Source: CAD feature listing. Evaluate the final solid. Frame: model axes, mm. A direction names the side the tool comes from. Round coordinates to 2 decimals unless told otherwise and drop trailing zeros. Write each loop counter-clockwise with the first axis right and the second up, starting at its lowest first coordinate (ties: lowest second). Pieces come first, ordered by that corner, then holes. Notation, with made-up numbers: M 35,-28 L 75,-28 A29 ccw 75,6 Z; hole C 20,75 d11. An arc over 180 degrees is marked long. Put each result on its own line as item: value. Start each with the question number.
```python
from build123d import *

# Parameters (mm, degrees)
F0_R     = 10.535173
F1_DEPTH = 40.894


with BuildPart() as f1:
    # F0 (on Front) → F1 (new body)
    with BuildSketch(Plane.XZ):
        with BuildLine():
            Line((-35.451322, 27.514845), (-11.27987, 27.514845))
            ThreePointArc((-11.27987, 27.514845), (-17.816037, 48.643776), (-35.141124, 62.391305))
            ThreePointArc((-35.141124, 62.391305), (-86.04097, 25.118193), (-30.793919, -5.342315))
            ThreePointArc((-30.793919, -5.342315), (-19.953258, 3.559245), (-13.152019, 15.827123))
            Line((-13.152019, 15.827123), (-42.462349, 15.827123))
            ThreePointArc((-42.462349, 15.827123), (-60.059173, 34.329486), (-35.451322, 27.514845))
        make_face()
        with BuildLine():
            ThreePointArc((-35.141124, 62.391305), (-17.816037, 48.643776), (-11.27987, 27.514845))
            Line((-11.27987, 27.514845), (11.076483, 27.514845))
            Line((11.076483, 27.514845), (11.076483, 15.827123))
            Line((11.076483, 15.827123), (-13.152019, 15.827123))
            ThreePointArc((-13.152019, 15.827123), (-19.953258, 3.559245), (-30.793919, -5.342315))
            Line((-30.793919, -5.342315), (52.946884, 16.285895))
            ThreePointArc((52.946884, 16.285895), (43.042984, 36.280636), (52.946884, 56.275376))
            Line((52.946884, 56.275376), (-35.141124, 62.391305))
        make_face()
        with BuildLine():
            ThreePointArc((93.313772, 36.280636), (79.334956, 58.804375), (52.946884, 56.275376))
            ThreePointArc((52.946884, 56.275376), (43.042984, 36.280636), (52.946884, 16.285895))
            ThreePointArc((52.946884, 16.285895), (79.334956, 13.756897), (93.313772, 36.280636))
        make_face()
        with Locations((68.178378, 36.280636)):
            Circle(F0_R, mode=Mode.SUBTRACT)
    extrude(amount=F1_DEPTH)


solid = f1.part
```
(1) Access query for faces 5 (the flat face through (11.076, -20, 22)), 6 (the flat face through (2, 0, 28)), 7 (the flat face through (10.49, -20.16, 5.32)). Directions: +Z, -Z, +X, -X, +Y, -Y. A direction counts if a zero-diameter tool reaches every point of the face in a straight line with its end or side. Return the directions, or none.
(2) Contact query for flat-ended pins moving along their axis: P1, Ø8, axis at x = -6, y = -28.5, coming from the +Z side; P2, Ø12.5, axis at x = -11, y = -30.5, coming from the +Z side; P3, Ø10, axis at x = -65, y = -32.5, coming from the -Z side. Output: stop coordinate, or through.
(3) Ray query, line 1 along X through (y, z) = (-30.5, 37); line 2 along X through (y, z) = (-39, 34.5); line 3 along Z through (x, y) = (1.5, -5). Return the intervals inside material, ascending.
(4) Section query A-A (y = -7). Return loops of the section in (x, z), and give its area (3 significant figures).
(5) Section query B-B (x = -44.5). Return loops of the section in (y, z), and give its area (3 significant figures).
(6) Section query C-C (z = 38.5). Return loops of the section in (x, y).
(7) Pull-direction query (Z, two-part tool) for faces 1 (the flat face through (2, -40.894, 28)), 2 (the cylindrical face through (-60.3, -20.16, 33.91)), 3 (the flat face through (-13, -20, 27.515)), 4 (the flat face through (9.52, -20.16, 59.29)); classes: +Z half, -Z half, draft (parallel to the pull), parting line (faces both ways), or undercut.
(8) Section query D-D (x = 61.5). Return loops of the section in (y, z), and give its area (3 significant figures).
Entries:
1. face 5: +Y, -Y
1. face 6: +Z, -Z, +X, -X, +Y
1. face 7: -Z, +Y, -Y
2. P1: z = 60.65
2. P2: z = 61.15
2. P3: z = -8.16
3. line 1: -84.9 to -57.95, -39.45 to 57.67, 78.69 to 93.3
3. line 2: -85.46 to -59.96, -37.44 to 57.79, 78.56 to 93.25
3. line 3: 3 to 15.83, 27.51 to 59.85
4. outline: M -35.14,62.39 A37.42 ccw long -30.79,-5.34 L 52.95,16.29 A25.14 ccw long 52.95,56.28 Z; hole M -42.46,15.83 L 11.08,15.83 L 11.08,27.51 L -35.45,27.51 A13.25 ccw long Z; hole C 68.18,36.28 d21.07
4. area: 8,230 mm2
5. outline: M -40.89,-9.67 L 0,-9.67 L 0,14.95 L -40.89,14.95 Z; M -40.89,40.08 L 0,40.08 L 0,64.7 L -40.89,64.7 Z
5. area: 2,010 mm2
6. outline: M -84.47,-40.89 L -56.1,-40.89 L -56.1,0 L -84.47,0 Z; M -41.29,-40.89 L 57.88,-40.89 L 57.88,0 L -41.29,0 Z; M 78.48,-40.89 L 93.22,-40.89 L 93.22,0 L 78.48,0 Z
7. face 1: draft
7. face 2: undercut
7. face 3: undercut
7. face 4: +Z half
8. outline: M -40.89,12.05 L 0,12.05 L 0,28.13 L -40.89,28.13 Z; M -40.89,44.43 L 0,44.43 L 0,60.51 L -40.89,60.51 Z
8. area: 1,320 mm2
